Work out the finished part from the listing and answer in its coordinate system (mm). Face numbers are marked on the shaded views. A direction names the side the tool comes from. Give positions to 0.01 mm unless a question says otherwise; leave off trailing zeros. Order: outer loops, then holes, each group sorted by start corner. A loop starts at its lowest first (then second) coordinate and runs counter-clockwise, first axis right, second up. Notation, with made-up numbers: (69, -10.5) -> (116, -10.5) arc R20 cw to (116, 14.5) -> close; hole circle Ø3 at (88, -38.75). An arc over 180 degrees is marked (long way). Answer as CSV lines item,"result". Start each with the question number.
1. For a pull along X with two mould halves and no side action, classify the marked faces 1, 2 and 3 as released by +X, released by -X, zero draft, split by the parting line, or undercut.
2. A cutting plane is placed at C-C (y = 1.5). State how many separate pieces and enclosed holes the cut face has, then the cut area to 3 significant figures.
3. A cutting plane is placed at D-D (x = 3.75). Give the vertices of the cut face in (y, z).
4. Flat-ended cylindrical pins translate along their axes: pin 1 (1.1 mm diameter, centred on x = 2, y = -0.5, fed in from -Z); pin 2 (2.5 mm diameter, centred on x = 3, y = 3.5, fed in from +Z); pin 3 (0.6 mm diameter, centred on y = 0.5, z = 4, fed in from -X). Find the tip coordinate at first contact, or state that the pin passes through.
5. A cutting plane is placed at A-A (x = -3). Give the vertices of the cut face in (y, z).
6. Find the intervals of material crossed by L1, parallel to X at y = -2.75, z = 3.25; L2, parallel to X at y = 4, z = 3.5; L3, parallel to X at y = 0.5, z = 2.5, in increasing order.
7. For the marked faces 4, 5, 6, 7 and 8, determine the directions among +Z, -Z, +X, -X, +Y, -Y from which every point of the face is accessible in a straight line to the end or side of a thin tool.
8. A cutting plane is placed at B-B (z = 5.5). Give the vertices of the cut face in (x, y), then the cut area to 3 significant figures.
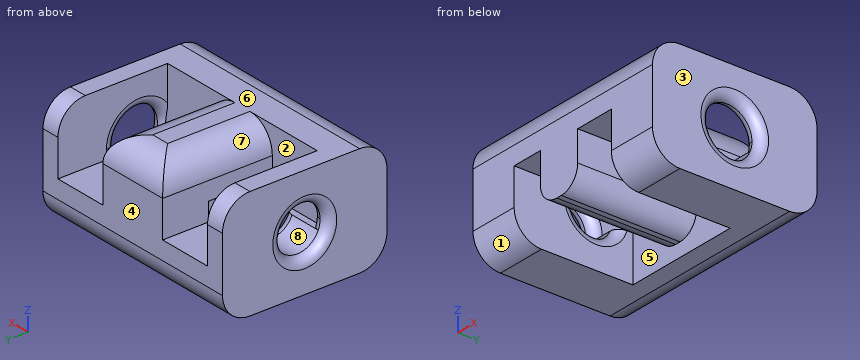
from build123d import *

# Parameters (mm, degrees)
F0_W          = 12
F0_H          = 9
F1_DEPTH      = 6
F2_W          = 3
F2_H          = 6
F3_DEPTH      = 3.5
F4_W          = 6.5
F4_H          = 6.5
F5_DEPTH      = 3.5
F6_R          = 1.35
F7_DEPTH      = 3
F8_R          = 1.25
F9_DEPTH      = 2.751
F10_R         = 1.5
F11_W         = 2.5
F11_H         = 6.5
F12_DEPTH     = 2.75
F13_R         = 1.1
F14_T8_ANGLE  = 247.5355258221
F14_T13_ANGLE = 74.7913514773
F14_T18_ANGLE = 254.8973081934
F14_T24_ANGLE = 80.8755372564
F14_T30_ANGLE = 260.9918579461


# Not quite as in the source:
# - a fillet or chamfer that OpenCascade refuses, or shapes differently, is made with other operations: its cross-section is extruded or revolved along the edge and cut away or added


with BuildPart() as f1:
    # F0 (on Top) → F1 (new body)
    with BuildSketch(Plane.XY):
        Rectangle(F0_W, F0_H)
    extrude(amount=F1_DEPTH)

    # F2 (on face) → F3 (cut)
    with BuildSketch(Plane.XY.offset(6)):
        with Locations((3.5, 1.5)):
            Rectangle(F2_W, F2_H)
        with Locations((-3.5, 1.5)):
            Rectangle(F2_W, F2_H)
    extrude(amount=-F3_DEPTH, mode=Mode.SUBTRACT)

    # F4 (on face) → F5 (cut)
    with BuildSketch(Plane(origin=(0, 0, 0), x_dir=(1, 0, 0), z_dir=(0, 0, -1))):
        with Locations((0, 1.25)):
            Rectangle(F4_W, F4_H)
    extrude(amount=-F5_DEPTH, mode=Mode.SUBTRACT)

    # F6 (on face) → F7 (cut)
    with BuildSketch(Plane.YZ.offset(6)):
        with Locations((0, 3)):
            Circle(F6_R)
    extrude(amount=-F7_DEPTH, mode=Mode.SUBTRACT)

    # F8 (on face) → F9 (cut, through all)
    with BuildSketch(Plane(origin=(-6, 0, 0), x_dir=(0, -1, 0), z_dir=(-1, 0, 0))):
        with Locations((0, 3)):
            Circle(F8_R)
    extrude(amount=-F9_DEPTH, mode=Mode.SUBTRACT)

    # F10
    f10_edges = [f1.edges().sort_by_distance(p)[0] for p in [
        (2, 1.5, 6),
        (-2, 1.5, 6),
        (0, -4.5, 6),
        (-4.625, -4.5, 0),
        (4.625, -4.5, 0),
        (0, 4.5, 0),
        (-5.5, 4.5, 6),
        (5.5, 4.5, 6),
        (0, 4.5, 6),
    ]]
    fillet(f10_edges, radius=F10_R)

    # F11 (on face) → F12 (join)
    with BuildSketch(Plane(origin=(0, 0, 3.5), x_dir=(1, 0, 0), z_dir=(0, 0, -1))):
        with Locations((-0.25, 1.25)):
            Rectangle(F11_W, F11_H)
    extrude(amount=F12_DEPTH)

    # F13
    f13_edges = [f1.edges().sort_by_distance(p)[0] for p in [
        (-1.5, -1.25, 0.75),
        (1, -1.25, 0.75),
    ]]
    fillet(f13_edges, radius=F13_R)

    # F14: fillet of radius 0.5 on 7 edges, made by hand

    # F14_s1 → F14_t2 (revolve, cut)
    with BuildSketch(Plane.XY.offset(3)):
        with BuildLine():
            ThreePointArc((6, 1.85), (5.8535533906, 1.4964466094), (5.5, 1.35))
            Line((5.5, 1.35), (6, 1.35))
            Line((6, 1.35), (6, 1.85))
        make_face()
    revolve(axis=Axis((6, 0, 3), (1, 0, 0)), mode=Mode.SUBTRACT)

    # F14_s3 → F14_t4 (revolve, cut)
    with BuildSketch(Plane.XY.offset(3)):
        with BuildLine():
            ThreePointArc((-6, -1.75), (-5.8535533906, -1.3964466094), (-5.5, -1.25))
            Line((-5.5, -1.25), (-6, -1.25))
            Line((-6, -1.25), (-6, -1.75))
        make_face()
    revolve(axis=Axis((-6, 0, 3), (-1, 0, 0)), mode=Mode.SUBTRACT)


with BuildPart() as f14_tool6:
    # F14_s7 → F14_t8 (revolve)
    with BuildSketch(Plane(origin=(0, -1.3861749524, 2.0731657713), x_dir=(1, 0, 0), z_dir=(0, -0.5558279796, 0.8312973338))):
        with BuildLine():
            ThreePointArc((-3.25, 3.4174839388), (-3.3964466094, 3.0639305482), (-3.75, 2.9174839388))
            Line((-3.75, 2.9174839388), (-3.25, 2.9174839388))
            Line((-3.25, 2.9174839388), (-3.25, 3.4174839388))
        make_face()
    revolve(axis=Axis((-3.25, 0, 3), (-1, 0, 0)), revolution_arc=F14_T8_ANGLE)

    split(bisect_by=Plane.XY.offset(3.5), keep=Keep.BOTTOM)


with BuildPart() as f1_1:
    add(f1.part)

    # F14_t5: cut F14_tool6
    add(f14_tool6.part, mode=Mode.SUBTRACT)


with BuildPart() as f14_tool11:
    # F14_s12 → F14_t13 (revolve)
    with BuildSketch(Plane(origin=(0, 0.7594411885, 0.2064587052), x_dir=(1, 0, 0), z_dir=(0, -0.9649769073, -0.2623348403))):
        with BuildLine():
            ThreePointArc((5.5, 1.5449307218), (5.1464466094, 1.3984841124), (5, 1.0449307218))
            Line((5, 1.0449307218), (5, 1.5449307218))
            Line((5, 1.5449307218), (5.5, 1.5449307218))
        make_face()
    revolve(axis=Axis((5, 0, 3), (1, 0, 0)), revolution_arc=F14_T13_ANGLE)

    split(bisect_by=Plane.XY.offset(2.5), keep=Keep.TOP)


with BuildPart() as f1_2:
    add(f1_1.part)

    # F14_t10: cut F14_tool11
    add(f14_tool11.part, mode=Mode.SUBTRACT)


with BuildPart() as f14_tool16:
    # F14_s17 → F14_t18 (revolve)
    with BuildSketch(Plane.XY.offset(3)):
        with BuildLine():
            ThreePointArc((5.5, 1.35), (5.1464466094, 1.4964466094), (5, 1.85))
            Line((5, 1.85), (5, 1.35))
            Line((5, 1.35), (5.5, 1.35))
        make_face()
    revolve(axis=Axis((5, 0, 3), (1, 0, 0)), revolution_arc=F14_T18_ANGLE)

    split(bisect_by=Plane.XZ.offset(1.5), keep=Keep.BOTTOM)

    split(bisect_by=Plane.XY.offset(2.5), keep=Keep.TOP)


with BuildPart() as f1_3:
    add(f1_2.part)

    # F14_t15: cut F14_tool16
    add(f14_tool16.part, mode=Mode.SUBTRACT)


with BuildPart() as f14_tool22:
    # F14_s23 → F14_t24 (revolve)
    with BuildSketch(Plane(origin=(0, -0.469718994, 0.0754425014), x_dir=(1, 0, 0), z_dir=(0, 0.9873461903, -0.1585796345))):
        with BuildLine():
            ThreePointArc((-5.5, -1.7120385709), (-5.1464466094, -1.5655919615), (-5, -1.2120385709))
            Line((-5, -1.2120385709), (-5, -1.7120385709))
            Line((-5, -1.7120385709), (-5.5, -1.7120385709))
        make_face()
    revolve(axis=Axis((-5, 0, 3), (-1, 0, 0)), revolution_arc=F14_T24_ANGLE)

    split(bisect_by=Plane.XZ.offset(1.5), keep=Keep.BOTTOM)

    split(bisect_by=Plane.XY.offset(2.5), keep=Keep.TOP)


with BuildPart() as f1_4:
    add(f1_3.part)

    # F14_t21: cut F14_tool22
    add(f14_tool22.part, mode=Mode.SUBTRACT)


with BuildPart() as f14_tool28:
    # F14_s29 → F14_t30 (revolve)
    with BuildSketch(Plane.XY.offset(3)):
        with BuildLine():
            ThreePointArc((-5.5, -1.25), (-5.1464466094, -1.3964466094), (-5, -1.75))
            Line((-5, -1.75), (-5, -1.25))
            Line((-5, -1.25), (-5.5, -1.25))
        make_face()
    revolve(axis=Axis((-5, 0, 3), (-1, 0, 0)), revolution_arc=F14_T30_ANGLE)

    split(bisect_by=Plane.XZ.offset(1.5), keep=Keep.BOTTOM)

    split(bisect_by=Plane.XY.offset(2.5), keep=Keep.TOP)


with BuildPart() as f1_5:
    add(f1_4.part)

    # F14_t27: cut F14_tool28
    add(f14_tool28.part, mode=Mode.SUBTRACT)


solid = f1_5.part
Answer sheet:
1,face 1,"zero draft"
1,face 2,"undercut"
1,face 3,"released by +X"
2,separate pieces,"3"
2,enclosed holes,"0"
2,area,"35.7 mm^2"
3,outline,"(-4.5, 1.5) arc R1.5 ccw to (-3, 0) -> (3, 0) arc R1.5 ccw to (4.5, 1.5) -> (4.5, 2.5) -> (1.25, 2.5) arc R1.35 cw to (-1.25, 2.5) -> (-1.5, 2.5) -> (-1.5, 6) -> (-3, 6) arc R1.5 ccw to (-4.5, 4.5) -> close"
4,pin 1,"stops at z = 3.5"
4,pin 2,"stops at z = 5.33"
4,pin 3,"stops at x = -5.87"
5,outline,"(-4.5, 3.5) -> (-1.5, 3.5) -> (-1.5, 6) -> (-3, 6) arc R1.5 ccw to (-4.5, 4.5) -> close; (2, 0) -> (3, 0) arc R1.5 ccw to (4.5, 1.5) -> (4.5, 2.5) -> (2, 2.5) -> close"
6,L1,"x = -6 to -3.25, -1.5 to 1, 3.25 to 6"
6,L2,"x = -6 to -5, -2 to 2, 5 to 6"
6,L3,"x = -1.5 to 1"
7,face 4,"+Z, -Z, +X, -X, +Y"
7,face 5,"-Z, -Y"
7,face 6,"+Z, +X, -X, +Y, -Y"
7,face 7,"+Z, +Y"
7,face 8,"-X"
8,outline,"(-6, -4.12) -> (6, -4.12) -> (6, 4.12) -> (5, 4.12) -> (5, -1.5) -> (1.62, -1.5) -> (1.62, 4.12) -> (-1.62, 4.12) -> (-1.62, -1.5) -> (-5, -1.5) -> (-5, 4.12) -> (-6, 4.12) -> close"
8,area,"60.8 mm^2"
